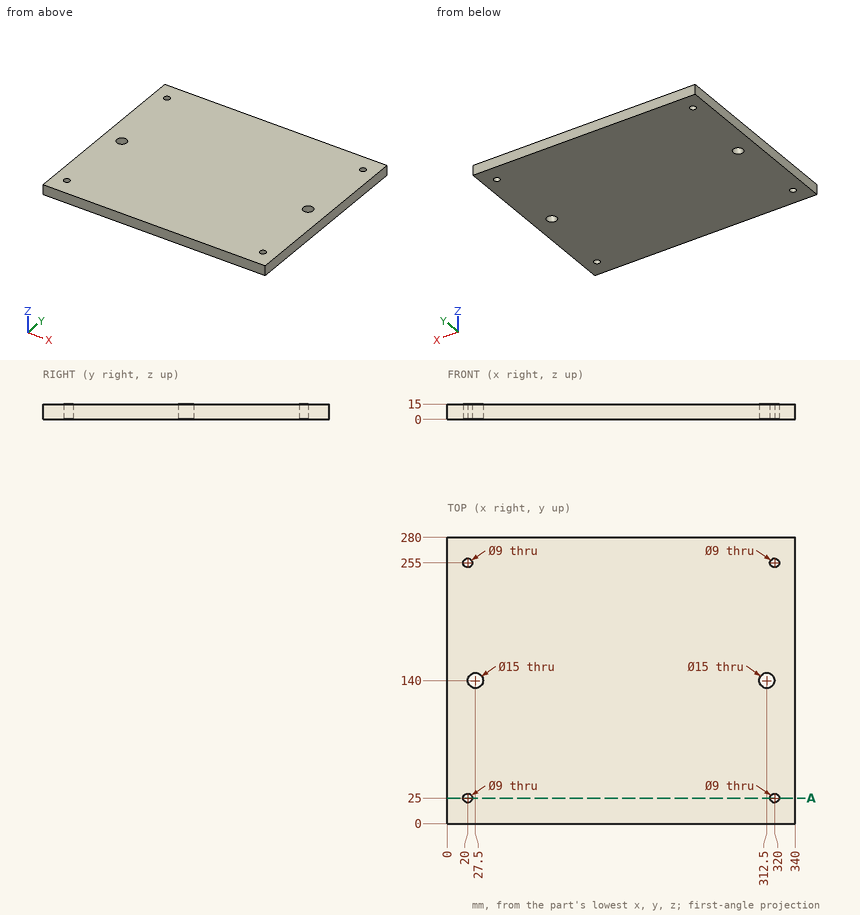
Drawing for the job (mm, zero at the part's lowest x, y, z). Coordinates: 2 decimals unless noted, no trailing zeros. Write each loop counter-clockwise with the first axis right and the second up, starting at its lowest first coordinate (ties: lowest second). Pieces come first, ordered by that corner, then holes. Notation, with made-up numbers: (7, -21.75) -> (39, -21.75) arc R17 ccw to (39, -16.75) -> close; hole circle Ø11 at (7.5, 25). An arc over 180 degrees is marked (long way). One line per item, written item: value. Start each with the question number.
1) Probe probe 1 along Y at (x, z) = (27.5, 4); probe 2 along X at (y, z) = (137, 11); probe 3 along Y at (x, z) = (33, 6.75). List the from-to ranges inside material, lowest first.
2) Flat gauge pin, fed straight in: pin 1 Ø7 at (x, y) = (20, 255) entering from -Z. Where does the tip first touch, or does it go through?
3) Slice it at A-A on y = 25. Write the cut outline in (x, z).
Answers follow:
1. probe 1: 0 to 132.5, 147.5 to 280
1. probe 2: 0 to 20.63, 34.37 to 305.63, 319.37 to 340
1. probe 3: 0 to 134.9, 145.1 to 280
2. pin 1: through
3. outline: (0, 0) -> (15.5, 0) -> (15.5, 15) -> (0, 15) -> close; (24.5, 0) -> (315.5, 0) -> (315.5, 15) -> (24.5, 15) -> close; (324.5, 0) -> (340, 0) -> (340, 15) -> (324.5, 15) -> close
